Geometry: final body of the model. Coordinates: model frame, mm. A direction names the side the tool comes from. Coordinates: 2 decimals unless noted, no trailing zeros. Write each loop counter-clockwise with the first axis right and the second up, starting at its lowest first coordinate (ties: lowest second). Pieces come first, ordered by that corner, then holes. Notation, with made-up numbers: M 2.25,18 L 47.25,18 A12 ccw 47.25,33 Z; hole C 69.5,39.5 d1. An arc over 180 degrees is marked long. Write item = value, one per line. Start each with the question number.
Item 1: Section A-A on x = 1063.5. Output: boundary loops of the cut face in (y, z).
Item 2: Section C-C on z = 1106.5. Output: boundary loops of the cut face in (x, y), plus the area to 3 significant figures.
Item 3: Section B-B on y = 161. Output: boundary loops of the cut face in (x, z).
Item 4: Ray query, L1, parallel to Z at x = 1428, y = 153; L2, parallel to X at y = 40, z = 1106.5; L3, parallel to Y at x = 1427.5, z = 1442. Return the intervals inside material, ascending. Write a range as [from, to].
Item 5: Reachability of faces 1 (the flat face through (1425, 450, 1221)), 2 (the flat face through (1450, 25, 621)), 3 (the flat face through (50, 475, 148)), 4 (the flat face through (75, 450, 1673)) from +Z, -Z, +X, -X, +Y, -Y: full face, straight path, thin tool, end or side. Return the list, or none.
Item 6: Pull-direction query (Z, two-part tool) for faces 5 (the flat face through (1450, 450, 1800)), 6 (the flat face through (740, 0, 1525)), 7 (the flat face through (1475, 450, 1221)); classes: +Z half, -Z half, draft (parallel to the pull), parting line (faces both ways), or undercut.
Item 7: Section D-D on y = 50.5. Give the number of separate pieces and of enclosed holes in the cut face, plus the area to 3 significant figures.
Item 8: First-contact query: pin 1 Ø25 at (x, z) = (41.5, 1691) entering from +Y; pin 2 Ø8 at (x, y) = (1274.5, 200) entering from -Z; pin 3 Ø1 at (x, y) = (158, 106) entering from +Z. Flat tips, straight axial feed; report the tip coordinate or a pass-through.
from build123d import *

# Parameters (mm, degrees)
F1_W      = 1500
F1_H      = 500
F2_DEPTH  = 50
F3_W      = 50
F3_H      = 50
F4_DEPTH  = 1800
F6_W      = 1500
F6_H      = 500
F7_DEPTH  = 50
F9_W      = 1500
F9_H      = 500
F10_DEPTH = 50


with BuildPart() as f2:
    # F1 (on offset) → F2 (new body)
    with BuildSketch(Plane.XY.offset(300)):
        with Locations((750, 250)):
            Rectangle(F1_W, F1_H)
    extrude(amount=F2_DEPTH)

    # F3 (on Top) → F4 (join)
    with BuildSketch(Plane.XY):
        with Locations((50, 50)):
            Rectangle(F3_W, F3_H)
        with Locations((1450, 50)):
            Rectangle(F3_W, F3_H)
        with Locations((1450, 450)):
            Rectangle(F3_W, F3_H)
        with Locations((50, 450)):
            Rectangle(F3_W, F3_H)
    extrude(amount=F4_DEPTH)

    # F6 (on offset) → F7 (join)
    with BuildSketch(Plane.XY.offset(900)):
        with Locations((750, 250)):
            Rectangle(F6_W, F6_H)
    extrude(amount=F7_DEPTH)

    # F9 (on offset) → F10 (join)
    with BuildSketch(Plane.XY.offset(1500)):
        with Locations((750, 250)):
            Rectangle(F9_W, F9_H)
    extrude(amount=F10_DEPTH)


solid = f2.part
Responses:
q1.outline = M 0,300 L 500,300 L 500,350 L 0,350 Z; M 0,900 L 500,900 L 500,950 L 0,950 Z; M 0,1500 L 500,1500 L 500,1550 L 0,1550 Z
q2.outline = M 25,25 L 75,25 L 75,75 L 25,75 Z; M 25,425 L 75,425 L 75,475 L 25,475 Z; M 1425,25 L 1475,25 L 1475,75 L 1425,75 Z; M 1425,425 L 1475,425 L 1475,475 L 1425,475 Z
q2.area = 10,000 mm²
q3.outline = M 0,300 L 1500,300 L 1500,350 L 0,350 Z; M 0,900 L 1500,900 L 1500,950 L 0,950 Z; M 0,1500 L 1500,1500 L 1500,1550 L 0,1550 Z
q4.L1 = [300, 350], [900, 950], [1500, 1550]
q4.L2 = [25, 75], [1425, 1475]
q4.L3 = [25, 75], [425, 475]
q5.face_1 = +Y, -Y
q5.face_2 = +X, -X, -Y
q5.face_3 = -Z, +X, -X, +Y
q5.face_4 = +Z, +Y, -Y
q6.face_5 = +Z half
q6.face_6 = draft
q6.face_7 = undercut
q7.separate_pieces = 1
q7.enclosed_holes = 2
q7.area = 390,000 mm²
q8.pin_1 = 475
q8.pin_2 = 300
q8.pin_3 = 1550
